Autodesk Inventor part; units mm, degrees
ref_plane "YZ Plane" through (0, 0, 0) normal (1, 0, 0) x (0, 1, 0)
ref_plane "XZ Plane" through (0, 0, 0) normal (0, 1, 0) x (-1, 0, 0)
ref_plane "XY Plane" through (0, 0, 0) normal (0, 0, 1) x (1, 0, 0)
sketch "Náčrt2" plane through (0, 0, 0) normal (1, 0, 0) x (0, 1, 0)
  line L0 (800, 400) -> (0, 400)
  line L1 (0, 400) -> (0, -400)
  line L2 (0, -400) -> (800, -400)
  line L3 (800, -400) -> (800, 400)
  point P0 (0, 0)
  point P1 (0, 0)
  dimension "d0" = 800
  dimension "d1" = 800
extrude "Vysunutí1" add sketch "Náčrt2" against normal blind 2.5
sketch "Náčrt3" plane through (-2.5, 797.5, 400) normal (0, 1, 0) x (-1, 0, 0)
  line L0 (0, -800) -> (0, 0)
  line L1 (0, 0) -> (-31.5, 0)
  line L2 (-31.5, 0) -> (-31.5, -800)
  line L3 (-31.5, -800) -> (0, -800)
edge flange "Obruba1" height 31.5 angle 90 thickness 2.5 bend radius 6 thickness toward (0, 1, 0) relief tear relief width 2.5 relief depth 1.25 corner gap 2.5 corner form 0 edges at (0, 800, 0) (0, 0, 0) wall of the first edge with corners at (-2.5, 797.5, -400) (-2.5, 797.5, 400) (29, 797.5, 400) (29, 797.5, -400)
bend "Ohyb1"
corner "Roh1"
equation "\"d4\" = ŠířkaVýštipu"
equation "\"d5\" = HloubkaVýštipu"
equation "\"d6\" = MinimálníZbytek"
equation "\"d7\" = PoloměrOhybu"
equation "\"d11\" = VelikostRohovéhoVýštipu"
equation "\"d12\" = VelikostMezery"
equation "\"d13\" = VelikostJacobihoPoloměru"
equation "\"PoloměrOhybu\" = Tloušťka"
equation "\"ŠířkaVýštipu\" = Tloušťka"
equation "\"HloubkaVýštipu\" = 0.5 * Tloušťka"
equation "\"MinimálníZbytek\" = 2 * Tloušťka"
equation "\"PřechodovýPoloměr\" = PoloměrOhybu"
equation "\"VelikostJacobihoPoloměru\" = PoloměrOhybu"
equation "\"VelikostMezery\" = Tloušťka"
properties part number "DD_KVD_002_02" material "Nerezová ocel"
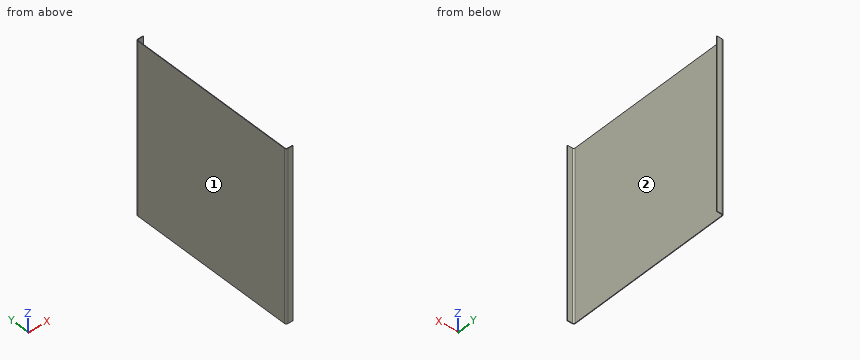
Source: CAD feature listing. Evaluate the final solid. Frame: model axes, mm. Face numbers are marked on the shaded views. A direction names the side the tool comes from. Give positions to 0.01 mm unless a question says otherwise; leave off trailing zeros. Write each loop counter-clockwise with the first axis right and the second up, starting at its lowest first coordinate (ties: lowest second). Pieces come first, ordered by that corner, then holes.
1. Section query A-A (x = 15). Return the cut outline in (y, z), then the cut area to 3 significant figures.
2. Section query B-B (z = 0). Return the cut outline in (x, y).
3. Section query C-C (y = 725.5). Return the cut outline in (x, z).
4. Access query for the marked faces 1 and 2. Directions: +Z, -Z, +X, -X, +Y, -Y. A direction counts if a zero-diameter tool reaches every point of the face in a straight line with its end or side. Return the directions, or none.
5. First-contact query: pin 1 (3 mm diameter, centred on y = 526.5, z = 201.5, fed in from +X); pin 2 (11.5 mm diameter, centred on x = 23, z = 11, fed in from -Y). Flat tips, straight axial feed; report the tip coordinate or a pass-through.
6. Material intervals for line 1 along Y through (x, z) = (27, 2); line 2 along X through (y, z) = (548.5, -191.5); line 3 along Y through (x, z) = (2.5, -105), sorted ascending.
Output values:
1. outline: (0, -400) - (2.5, -400) - (2.5, 400) - (0, 400) - close; (797.5, -400) - (800, -400) - (800, 400) - (797.5, 400) - close
1. area: 4,000 mm2
2. outline: (-2.5, 8.5) arc R8.5 ccw to (6, 0) - (29, 0) - (29, 2.5) - (6, 2.5) arc R6 cw to (0, 8.5) - (0, 791.5) arc R6 cw to (6, 797.5) - (29, 797.5) - (29, 800) - (6, 800) arc R8.5 ccw to (-2.5, 791.5) - close
3. outline: (-2.5, -400) - (0, -400) - (0, 400) - (-2.5, 400) - close
4. face 1: +Z, -Z, -X, +Y, -Y
4. face 2: +Z, -Z, +X
5. pin 1: stops at x = 0
5. pin 2: stops at y = 0
6. line 1: y = 0 to 2.5, 797.5 to 800
6. line 2: x = -2.5 to 0
6. line 3: y = 0.75 to 3.63, 796.37 to 799.25
